```python
from build123d import *

# Parameters (mm, degrees)
SKETCH_1_W      = 69
SKETCH_1_H      = 37
EXTRUDE_1_DEPTH = 18.8
FILLET_1_R      = 5


with BuildPart() as part:
    # 草图1 → 凸台-拉伸1 (new body)
    with BuildSketch(Plane(origin=(0, 0, 0), x_dir=(1, 0, 0), z_dir=(0, 1, 0))):
        Rectangle(SKETCH_1_W, SKETCH_1_H)
    extrude(amount=EXTRUDE_1_DEPTH)

    # 圆角1
    fillet_1_edges = [part.edges().sort_by_distance(p)[0] for p in [
        (0, 18.8, 18.5),
        (0, 0, 18.5),
        (0, 0, -18.5),
        (0, 18.8, -18.5),
    ]]
    fillet(fillet_1_edges, radius=FILLET_1_R)


solid = part.part
```
For this review, take the finished solid that the model builds, in its own axes (mm). Give positions to 0.01 mm unless a question says otherwise; leave off trailing zeros. Write each loop counter-clockwise with the first axis right and the second up, starting at its lowest first coordinate (ties: lowest second). Pieces come first, ordered by that corner, then holes. Notation, with made-up numbers: M -35,-6.75 L -15,-6.75 A15 ccw -15,22.25 Z; hole C 21,5 d5. An arc over 180 degrees is marked long. One line per item, written item: value.
1) Take a section at B-B, the plane y = 16. Write out the cut boundary in (x, z).
Results are:
outline: M -34.5,-17.99 L 34.5,-17.99 L 34.5,17.99 L -34.5,17.99 Z
2) Take a section at C-C, the plane z = 16. Write out the cut boundary in (x, y), then the cut area to 3 significant figures.
Results are:
outline: M -34.5,0.67 L 34.5,0.67 L 34.5,18.13 L -34.5,18.13 Z
area: 1,200 mm²
3) For line 1 (Z direction, x = -21, y = 15); line 2 (Z direction, x = -4.5, y = 17.5); line 3 (Y direction, x = 19.5, z = -16), list the stretches that pass through material, from the lowest coordinate up. Write a range as from..to.
Results are:
line 1: z = -18.35..18.35
line 2: z = -16.86..16.86
line 3: y = 0.67..18.13
4) The part is to be moulded in two halves that separate along X. For faces 1 (the flat face through (-34.5, 9, 0)), 2 (the flat face through (0, 0, 0)), 3 (the flat face through (34.5, 9, 0)), say which applies: +X half, -X half, draft (parallel to the pull), parting line (faces both ways), or undercut.
Results are:
face 1: -X half
face 2: draft
face 3: +X half
5) Take a section at A-A, the plane x = 10.5. Write out the cut boundary in (y, z), then the cut area to 3 significant figures.
Results are:
outline: M 0,-13.5 A5 ccw 5,-18.5 L 13.8,-18.5 A5 ccw 18.8,-13.5 L 18.8,13.5 A5 ccw 13.8,18.5 L 5,18.5 A5 ccw 0,13.5 Z
area: 674 mm²
